Check sheet for the modelled part. Datum: model origin and axes. Units: mm. Face numbers are marked on the shaded views. A direction names the side the tool comes from. Give positions to 0.01 mm unless a question says otherwise; leave off trailing zeros. Write each loop counter-clockwise with the first axis right and the second up, starting at its lowest first coordinate (ties: lowest second). Pieces come first, ordered by that corner, then holes. Notation, with made-up numbers: M -9,19 L 29,19 A15 ccw 29,39 Z; hole C -16,83.5 d5. An arc over 180 degrees is marked long. Write item = value, one per line. Start each with the question number.
1) Set-up check for the marked faces 1, 2 and 3: record each of +Z, -Z, +X, -X, +Y, -Y from which the full face is reachable in a straight line by a thin tool's end or side.
2) Sectioned sample at C-C, the plane y = -22. Record the cut outline in (x, z), then the cut area to 3 significant figures.
3) Scan lines: L1, parallel to X at y = -22, z = 2.1; L2, parallel to Z at x = 1, y = 16.5; L3, parallel to Y at x = -40, z = 1.2. Record each from-to range of solid material in increasing order.
4) Gauge pin test, flat ends, axial feed: pin 1 (1.6 mm diameter, centred on x = 5, y = 36, fed in from +Z); pin 2 (5 mm diameter, centred on x = 7.5, y = 28, fed in from +Z); pin 3 (4.5 mm diameter, centred on y = 8.5, z = 2.5, fed in from -X). Record the tip position at first contact, or that the pin passes through.
5) Sectioned sample at B-B, the plane z = -18.5. Record the cut outline in (x, y).
6) Sectioned sample at D-D, the plane z = -4. Record the cut outline in (x, y).
7) Sectioned sample at A-A, the plane x = -40. Record the cut outline in (y, z).
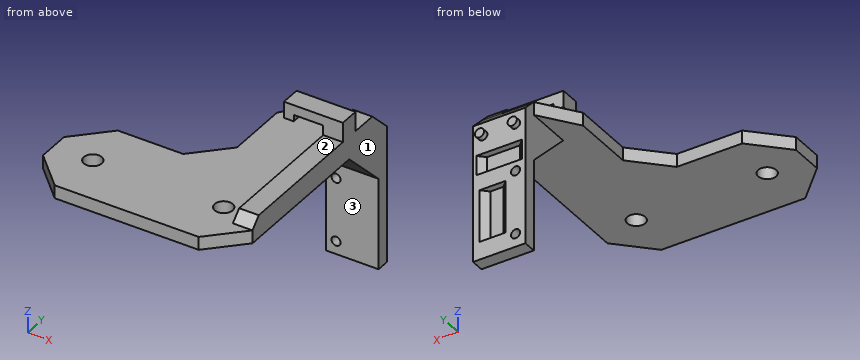
from build123d import *

# Parameters (mm, degrees)
SKETCH1_W           = 24
SKETCH1_H           = 74
BOSS_EXTRUDE1_DEPTH = 4
SKETCH3_W           = 24
SKETCH3_H           = 4
BOSS_EXTRUDE2_DEPTH = 42
CHAMFER1_SIZE       = 14
CHAMFER2_SIZE       = 4
SKETCH4_W           = 8
SKETCH4_H           = 42
CUT_EXTRUDE3_DEPTH  = 30
SKETCH5_R           = 1.4
BOSS_EXTRUDE3_DEPTH = 1.6
CUT_EXTRUDE4_REACH  = 87.93
SKETCH6_R           = 1.4
BOSS_EXTRUDE4_DEPTH = 6
CUT_EXTRUDE6_REACH  = 60.292
SKETCH11_W          = 40
SKETCH11_H          = 30
BOSS_EXTRUDE6_DEPTH = 4
CUT_EXTRUDE2_REACH  = 79.188
SKETCH2_R           = 2.75
CHAMFER3_SIZE       = 10
SKETCH12_W          = 3
SKETCH12_H          = 60
BOSS_EXTRUDE7_DEPTH = 6
CHAMFER4_SIZE       = 3
SKETCH13_W          = 4
SKETCH13_H          = 16
SKETCH13_W_2        = 10
SKETCH13_H_2        = 6
CUT_EXTRUDE7_DEPTH  = 2
CHAMFER5_SIZE       = 2


with BuildPart() as part:
    # Sketch1 → Boss-Extrude1 (new body)
    with BuildSketch(Plane.XY):
        Rectangle(SKETCH1_W, SKETCH1_H)
    extrude(amount=BOSS_EXTRUDE1_DEPTH)

    # Sketch3 → Boss-Extrude2 (add)
    with BuildSketch(Plane.XY):
        with Locations((0, 35)):
            Rectangle(SKETCH3_W, SKETCH3_H)
    extrude(amount=-BOSS_EXTRUDE2_DEPTH)

    # Chamfer1
    chamfer1_edges = [part.edges().sort_by_distance(p)[0] for p in [
        (0, 33, 0),
    ]]
    chamfer(chamfer1_edges, length=CHAMFER1_SIZE)

    # Chamfer2
    chamfer2_edges = [part.edges().sort_by_distance(p)[0] for p in [
        (0, 37, 4),
    ]]
    chamfer(chamfer2_edges, length=CHAMFER2_SIZE)

    # Sketch4 → Cut-Extrude3 (cut)
    with BuildSketch(Plane(origin=(0, 37, 0), x_dir=(1, 0, 0), z_dir=(0, 1, 0))):
        with Locations((-8, 21)):
            Rectangle(SKETCH4_W, SKETCH4_H)
    extrude(amount=-CUT_EXTRUDE3_DEPTH, mode=Mode.SUBTRACT)

    # Sketch5 → Boss-Extrude3 (add)
    with BuildSketch(Plane(origin=(0, 37, 0), x_dir=(1, 0, 0), z_dir=(0, 1, 0))):
        with Locations(Location((-1, 4, 0), (0, 0, 90))):
            Circle(SKETCH5_R)
        with Locations(Location((9, 4, 0), (0, 0, 90))):
            Circle(SKETCH5_R)
    extrude(amount=BOSS_EXTRUDE3_DEPTH)

    # Sketch6 → Cut-Extrude4 (cut, up to next)
    with BuildSketch(Plane(origin=(0, 37, 0), x_dir=(1, 0, 0), z_dir=(0, 1, 0)), mode=Mode.PRIVATE) as cut_extrude4_sk1:
        with Locations(Location((-1, 18.5, 0), (0, 0, 270))):
            Circle(SKETCH6_R)
    cut_extrude4_tool1 = extrude(cut_extrude4_sk1.sketch, amount=-CUT_EXTRUDE4_REACH, mode=Mode.PRIVATE) & part.part
    # Sketch6 → Cut-Extrude4 (cut, up to next)
    with BuildSketch(Plane(origin=(0, 37, 0), x_dir=(1, 0, 0), z_dir=(0, 1, 0)), mode=Mode.PRIVATE) as cut_extrude4_sk2:
        with Locations(Location((-1, 38, 0), (0, 0, 270))):
            Circle(SKETCH6_R)
    cut_extrude4_tool2 = extrude(cut_extrude4_sk2.sketch, amount=-CUT_EXTRUDE4_REACH, mode=Mode.PRIVATE) & part.part
    add(cut_extrude4_tool1.solids().sort_by_distance((-1, 37, -18.5))[0], mode=Mode.SUBTRACT)
    add(cut_extrude4_tool2.solids().sort_by_distance((-1, 37, -38))[0], mode=Mode.SUBTRACT)

    # Sketch7 → Boss-Extrude4 (add)
    with BuildSketch(Plane(origin=(0, 22, 0), x_dir=(1, 0, 0), z_dir=(0, 1, 0))):
        Polygon((12, -4), (12, -13), (-6, -13), (-6, -8), (-3, -8), (-3, -10), (6, -10), (6, -4), align=None)
    extrude(amount=-BOSS_EXTRUDE4_DEPTH)

    # Sketch9 → Cut-Extrude6 (cut, up to next)
    with BuildSketch(Plane.XY, mode=Mode.PRIVATE) as cut_extrude6_sk1:
        Polygon((-4, 37), (-4, 33), (-12, 22), (-12, 37), align=None)
    cut_extrude6_tool1 = extrude(cut_extrude6_sk1.sketch, amount=CUT_EXTRUDE6_REACH, mode=Mode.PRIVATE) & part.part
    add(cut_extrude6_tool1.solids().sort_by_distance((-8.77193, 31.719298, 0))[0], mode=Mode.SUBTRACT)

    # Sketch11 → Boss-Extrude6 (add)
    with BuildSketch(Plane.XY):
        with Locations((-32, -22)):
            Rectangle(SKETCH11_W, SKETCH11_H)
    extrude(amount=BOSS_EXTRUDE6_DEPTH)

    # Sketch2 → Cut-Extrude2 (cut, up to next)
    with BuildSketch(Plane.XY, mode=Mode.PRIVATE) as cut_extrude2_sk1:
        with Locations((0, -22)):
            Circle(SKETCH2_R)
    cut_extrude2_tool1 = extrude(cut_extrude2_sk1.sketch, amount=CUT_EXTRUDE2_REACH, mode=Mode.PRIVATE) & part.part
    # Sketch2 → Cut-Extrude2 (cut, up to next)
    with BuildSketch(Plane.XY, mode=Mode.PRIVATE) as cut_extrude2_sk2:
        with Locations((-40, -22)):
            Circle(SKETCH2_R)
    cut_extrude2_tool2 = extrude(cut_extrude2_sk2.sketch, amount=CUT_EXTRUDE2_REACH, mode=Mode.PRIVATE) & part.part
    add(cut_extrude2_tool1.solids().sort_by_distance((0, -22, 0))[0], mode=Mode.SUBTRACT)
    add(cut_extrude2_tool2.solids().sort_by_distance((-40, -22, 0))[0], mode=Mode.SUBTRACT)

    # Chamfer3
    chamfer3_edges = [part.edges().sort_by_distance(p)[0] for p in [
        (-12, -7, 2),
        (-52, -37, 2),
        (-52, -7, 2),
        (12, -37, 2),
    ]]
    chamfer(chamfer3_edges, length=CHAMFER3_SIZE)

    # Sketch12 → Boss-Extrude7 (add)
    with BuildSketch(Plane(origin=(12, 0, 0), x_dir=(0, 0, -1), z_dir=(1, 0, 0))):
        with Locations((-5.5, 3)):
            Rectangle(SKETCH12_W, SKETCH12_H)
    extrude(amount=-BOSS_EXTRUDE7_DEPTH)

    # Chamfer4
    chamfer4_edges = [part.edges().sort_by_distance(p)[0] for p in [
        (9, 33, 7),
        (9, -27, 7),
    ]]
    chamfer(chamfer4_edges, length=CHAMFER4_SIZE - 0.0001)  # a hair under: the kernel refuses the full size

    # Sketch13 → Cut-Extrude7 (cut)
    with BuildSketch(Plane(origin=(0, 37, 0), x_dir=(1, 0, 0), z_dir=(0, 1, 0))):
        with Locations((6, 28.5)):
            Rectangle(SKETCH13_W, SKETCH13_H)
        with Locations((4, 12.5)):
            Rectangle(SKETCH13_W_2, SKETCH13_H_2)
    extrude(amount=-CUT_EXTRUDE7_DEPTH, mode=Mode.SUBTRACT)

    # Chamfer5
    chamfer5_edges = [part.edges().sort_by_distance(p)[0] for p in [
        (4, 37, -28.5),
        (-1, 37, -12.5),
        (9, 37, -12.5),
        (8, 37, -28.5),
    ]]
    chamfer(chamfer5_edges, length=CHAMFER5_SIZE - 0.0001)  # a hair under: the kernel refuses the full size


solid = part.part
Data:
q1.face_1 = +Z, -Z, +X, +Y, -Y
q1.face_2 = +Z, +X, -X, -Y
q1.face_3 = -Z, +X, -X, -Y
q2.outline = M -52,0 L -42.75,0 L -42.75,4 L -52,4 Z; M -37.25,0 L -2.75,0 L -2.75,4 L -37.25,4 Z; M 2.75,0 L 12,0 L 12,7 L 6,7 L 6,4 L 2.75,4 Z
q2.area = 230 mm2
q3.L1 = -52 to -42.75, -37.25 to -2.75, 2.75 to 12
q3.L2 = 0 to 4, 10 to 13
q3.L3 = -37 to -24.75, -19.25 to -7
q4.pin_1 = 1.8
q4.pin_2 = 7
q4.pin_3 = -12
q5.outline = M -4,33 L -2.4,33 L -2.4,37 L -4,37 Z; M 0.4,33 L 12,33 L 12,37 L 0.4,37 Z
q6.outline = M -4,23 L 12,23 L 12,37 L 10.4,37 L 10.4,38.6 L 7.6,38.6 L 7.6,37 L 0.4,37 L 0.4,38.6 L -2.4,38.6 L -2.4,37 L -4,37 Z
q7.outline = M -37,0 L -24.75,0 L -24.75,4 L -37,4 Z; M -19.25,0 L -7,0 L -7,4 L -19.25,4 Z
